from build123d import *

# Parameters (mm, degrees)
F1_DEPTH = 609.6
F3_R     = 1.27
F4_DEPTH = 3.81
F6_DEPTH = 3.81
F7_R     = 1.27
F8_R     = 1.27


with BuildPart() as f1:
    # F0 (on Front) → F1 (new body)
    with BuildSketch(Plane.XZ):
        Polygon((0, 50.8), (0, 0), (50.8, 0), (50.8, 3.175), (3.175, 3.175), (3.175, 50.8), align=None)
    extrude(amount=F1_DEPTH)

    # F3
    f3_edges = [f1.edges().sort_by_distance(p)[0] for p in [
        (3.175, -304.8, 50.8),
        (0, -304.8, 50.8),
        (1.5875, 0, 50.8),
        (1.5875, -609.6, 50.8),
    ]]
    fillet(f3_edges, radius=F3_R)

    # F2 (on face) → F4 (cut)
    with BuildSketch(Plane.XY.offset(3.175)):
        Polygon((50.8, 0), (3.175, 0), (50.8, -47.625), align=None)
    extrude(amount=-F4_DEPTH, mode=Mode.SUBTRACT)

    # F5 (on face) → F6 (cut)
    with BuildSketch(Plane.XY.offset(3.175)):
        Polygon((50.8, -561.975), (3.175, -609.6), (50.8, -609.6), align=None)
    extrude(amount=-F6_DEPTH, mode=Mode.SUBTRACT)

    # F7
    f7_edges = [f1.edges().sort_by_distance(p)[0] for p in [
        (50.8, -304.8, 3.175),
        (50.8, -561.975, 1.5875),
        (50.8, -304.8, 0),
        (50.8, -47.625, 1.5875),
    ]]
    fillet(f7_edges, radius=F7_R)

    # F8
    f8_edges = [f1.edges().sort_by_distance(p)[0] for p in [
        (0, -304.8, 0),
    ]]
    fillet(f8_edges, radius=F8_R)


solid = f1.part
The listing builds one solid part. Answer for the finished solid, in the listing's coordinates (mm). A direction names the side the tool comes from. Round coordinates to 2 decimals unless told otherwise and drop trailing zeros. Write each loop counter-clockwise with the first axis right and the second up, starting at its lowest first coordinate (ties: lowest second). Pieces come first, ordered by that corner, then holes. Notation, with made-up numbers: M -7.5,0 L 12.5,0 A29 ccw 12.5,29 Z; hole C 62,-16 d9. An arc over 180 degrees is marked long. Write each question's results on one line, items separated by ' | '. Start each with the question number.
Item 1: Find section B-B on z = 29.5. Write down the section's boundary in (x, y) (3 decimals), and give its area (3 significant figures).
Item 2: Find section A-A on y = -159. Write down the section's boundary in (x, z) (3 decimals), and give its area (3 significant figures).
Item 3: Which of the six approach directions +Z, -Z, +X, -X, +Y, -Y give full straight-line access (tool end or side, diameter ignored) to faces 1 (the flat face through (26.471, -23.296, 1.61)), 2 (the flat face through (27, -301, 3.175))?
Item 4: A straight line is drawn through the part: probe 1 along Z at (x, y) = (37, -238) (3 decimals). Find the intervals that lie inside material, in ascending order.
Item 5: Given pin 1 Ø5 at (x, y) = (18, -146) entering from +Z (3 decimals); pin 2 Ø4 at (y, z) = (-437.5, 38.5) entering from +X (3 decimals), each flat-ended and moving along its own axis, determine where each tip first touches the part or whether it passes through.
Item 6: Find section C-C on x = 17. Write down the section's boundary in (y, z) (3 decimals).
Answer block:
1) outline: M 0,-609.6 L 3.175,-609.6 L 3.175,0 L 0,0 Z | area: 1,940 mm²
2) outline: M 0,1.27 A1.27 ccw 1.27,0 L 49.53,0 A1.27 ccw 50.8,1.27 L 50.8,1.905 A1.27 ccw 49.53,3.175 L 3.175,3.175 L 3.175,49.53 A1.27 ccw 1.905,50.8 L 1.27,50.8 A1.27 ccw 0,49.53 Z | area: 311 mm²
3) face 1: +Z, -Z, +X, +Y | face 2: +Z, +X, +Y, -Y
4) probe 1: z = 0 to 3.175
5) pin 1: stops at z = 3.175 | pin 2: stops at x = 3.175
6) outline: M -595.775,0 L -13.825,0 L -13.825,3.175 L -595.775,3.175 Z
